from build123d import *

# Parameters (mm, degrees)
EXTRUDE_1_DEPTH     = 25
SKETCH_2_R          = 1.1
CUT_EXTRUDE_1_DEPTH = 3
CUT_EXTRUDE_START   = -3
SKETCH_3_R          = 1.1
CUT_EXTRUDE_2_DEPTH = 3


with BuildPart() as part:
    # 草图1 → 凸台-拉伸1 (new body)
    with BuildSketch(Plane.XY):
        Polygon((1.732050808, 0), (0.866025404, 1.5), (-0.866025404, 1.5), (-1.732050808, 0), (-0.866025404, -1.5), (0.866025404, -1.5), align=None)
    extrude(amount=EXTRUDE_1_DEPTH)

    # 草图2 → 切除-拉伸1 (cut)
    with BuildSketch(Plane.XY.offset(25)):
        Circle(SKETCH_2_R)
    extrude(amount=-CUT_EXTRUDE_1_DEPTH, mode=Mode.SUBTRACT)

    # 草图3 → 切除-拉伸2 (cut)
    with BuildSketch(Plane(origin=(0, 0, 0), x_dir=(-1, 0, 0), z_dir=(0, 0, -1)).offset(CUT_EXTRUDE_START)):
        with Locations(Location((0, 0, 0), (0, 0, 180))):
            Circle(SKETCH_3_R)
    extrude(amount=CUT_EXTRUDE_2_DEPTH, mode=Mode.SUBTRACT)


solid = part.part
Design review of the part built by this model. Coordinates are the model's own, in mm. A direction names the side the tool comes from. Round coordinates to 2 decimals unless told otherwise and drop trailing zeros. Loops run counter-clockwise (first coordinate to the right, second up) from the corner with the lowest first, then second, coordinate; pieces in that order, holes last. Notation, with made-up numbers: M 68,-8.5 L 73,-8.5 A21 ccw 73,19.5 Z; hole C 69,44 d9. An arc over 180 degrees is marked long. Answer as a JSON object with one key per item and string values.
Item 1: Wall thickness on L1, parallel to Y at x = 0, z = 24.3; L2, parallel to Z at x = 0.55, y = -0.5; L3, parallel to X at y = -0.4, z = 3.5: over which ranges is each line inside the solid? List them lowest first. Write a range as from..to.
Answer sheet:
{"L1": "y = -1.5..-1.1, 1.1..1.5", "L2": "z = 3..22", "L3": "x = -1.5..1.5"}
Item 2: We need section A-A on x = 0. Give the boundary of the cut face in (y, z), and give its area (3 significant figures).
Answer sheet:
{"outline": "M -1.5,0 L -1.1,0 L -1.1,3 L 1.1,3 L 1.1,0 L 1.5,0 L 1.5,25 L 1.1,25 L 1.1,22 L -1.1,22 L -1.1,25 L -1.5,25 Z", "area": "61.8 mm^2"}
Item 3: Machinability: for faces 1 (the cylindrical face through (-0.14, -1.09, 1.52)), 2 (the cylindrical face through (1.05, 0.33, 23.52)), 3 (the flat face through (-1.305, -0.74, 12.325)), which of the approach directions +Z, -Z, +X, -X, +Y, -Y give a long, thin tool a straight path to every point of the face, cutting with its end or side? Answer none if there is none.
Answer sheet:
{"face 1": "-Z", "face 2": "+Z", "face 3": "+Z, -Z, -X, -Y"}
Item 4: The part is to be moulded in two halves that separate along Y. For faces 4 (the flat face through (0.75, 1.02, 25)), 5 (the flat face through (0, 1.5, 12)), 6 (the flat face through (0, 0, 3)), say which applies: pulls with the +Y half, pulls with the -Y half, needs draft (parallel to the pull), parting line crosses it, or undercut.
Answer sheet:
{"face 4": "needs draft", "face 5": "pulls with the +Y half", "face 6": "undercut"}
Item 5: We need section C-C on y = -0.55. Give the boundary of the cut face in (x, z), and give its area (3 significant figures).
Answer sheet:
{"outline": "M -1.41,0 L -0.95,0 L -0.95,3 L 0.95,3 L 0.95,0 L 1.41,0 L 1.41,25 L 0.95,25 L 0.95,22 L -0.95,22 L -0.95,25 L -1.41,25 Z", "area": "59.3 mm^2"}
Item 6: Clearance check with flat-ended pins moving along their axes: P1, Ø1.8, axis at x = 0, y = 0, coming from the +Z side; P2, Ø1.8, axis at x = -0.5, y = 0, coming from the -Z side. State where each tip first meets the part, or that it passes through.
Answer sheet:
{"P1": "stops at z = 22", "P2": "stops at z = 0"}
Item 7: We need section B-B on z = 10.25. Give the boundary of the cut face in (x, y), and give its area (3 significant figures).
Answer sheet:
{"outline": "M -1.73,0 L -0.87,-1.5 L 0.87,-1.5 L 1.73,0 L 0.87,1.5 L -0.87,1.5 Z", "area": "7.79 mm^2"}
